```python
from build123d import *

# Parameters (mm, degrees)
BOSS_EXTRUDE1_DEPTH     = 56
SKETCH2_R               = 20
BOSS_EXTRUDE2_DEPTH     = 2
SKETCH4_R               = 20
BOSS_EXTRUDE3_DEPTH     = 2
SKETCH5_R               = 2.5
CUT_EXTRUDE1_DEPTH      = 11
SKETCH6_R               = 2.5
CUT_EXTRUDE2_DEPTH      = 11
CUT_EXTRUDE3_DEPTH      = 147.710599481
CUT_EXTRUDE3_DEPTH_BACK = 147.710599481
SKETCH7_R               = 11
SKETCH8_R               = 11
CUT_EXTRUDE4_DEPTH      = 51


with BuildPart() as part:
    # Sketch1 → Boss-Extrude1 (new body)
    with BuildSketch(Plane.XY):
        Polygon((-52, 0), (52, 0), (52, -56), (28, -56), (28, -80), (-28, -80), (-28, -56), (-52, -56), align=None)
    extrude(amount=BOSS_EXTRUDE1_DEPTH)

    # Sketch2 → Boss-Extrude2 (add)
    with BuildSketch(Plane(origin=(52, 0, 0), x_dir=(0, 0, -1), z_dir=(1, 0, 0))):
        with Locations(Location((-28, -28, 0), (0, 0, 90))):
            Circle(SKETCH2_R)
    boss_extrude2 = extrude(amount=BOSS_EXTRUDE2_DEPTH)

    # Mirror1: Boss-Extrude2 across plane
    add(boss_extrude2.mirror(Plane(origin=(0, 0, 0), x_dir=(0, 0, 1), z_dir=(1, 0, 0))))

    # Sketch4 → Boss-Extrude3 (add)
    with BuildSketch(Plane.XZ.offset(80)):
        with Locations(Location((0, 28, 0), (0, 0, 270))):
            Circle(SKETCH4_R)
    extrude(amount=BOSS_EXTRUDE3_DEPTH)

    # Sketch5 → Cut-Extrude1 (cut)
    with BuildSketch(Plane(origin=(52, 0, 0), x_dir=(0, 0, -1), z_dir=(1, 0, 0))):
        with Locations(Location((-50, -6, 0), (0, 0, 90))):
            Circle(SKETCH5_R)
        with Locations(Location((-50, -50, 0), (0, 0, 90))):
            Circle(SKETCH5_R)
        with Locations(Location((-6, -50, 0), (0, 0, 90))):
            Circle(SKETCH5_R)
        with Locations(Location((-6, -6, 0), (0, 0, 90))):
            Circle(SKETCH5_R)
    cut_extrude1 = extrude(amount=-CUT_EXTRUDE1_DEPTH, mode=Mode.SUBTRACT)

    # Mirror2: Cut-Extrude1 across plane
    add(cut_extrude1.mirror(Plane(origin=(0, 0, 0), x_dir=(0, 0, 1), z_dir=(1, 0, 0))), mode=Mode.SUBTRACT)

    # Sketch6 → Cut-Extrude2 (cut)
    with BuildSketch(Plane.XZ.offset(80)):
        with Locations(Location((-22, 50, 0), (0, 0, 270))):
            Circle(SKETCH6_R)
        with Locations(Location((22, 50, 0), (0, 0, 270))):
            Circle(SKETCH6_R)
        with Locations(Location((22, 6, 0), (0, 0, 270))):
            Circle(SKETCH6_R)
        with Locations(Location((-22, 6, 0), (0, 0, 270))):
            Circle(SKETCH6_R)
    extrude(amount=-CUT_EXTRUDE2_DEPTH, mode=Mode.SUBTRACT)

    # Sketch7 → Cut-Extrude3 (cut, two sides: drawn at the far end of the back side and taken through both)
    with BuildSketch(Plane.ZY.offset(54).offset(-CUT_EXTRUDE3_DEPTH_BACK)):
        with Locations(Location((28, -28, 0), (0, 0, 270))):
            Circle(SKETCH7_R)
    extrude(amount=CUT_EXTRUDE3_DEPTH + CUT_EXTRUDE3_DEPTH_BACK, mode=Mode.SUBTRACT)

    # Sketch8 → Cut-Extrude4 (cut)
    with BuildSketch(Plane.XZ.offset(82)):
        with Locations(Location((0, 28, 0), (0, 0, 270))):
            Circle(SKETCH8_R)
    extrude(amount=-CUT_EXTRUDE4_DEPTH, mode=Mode.SUBTRACT)


solid = part.part
```
For this review, take the finished solid that the model builds, in its own axes (mm). A direction names the side the tool comes from. Round coordinates to 2 decimals unless told otherwise and drop trailing zeros. Write each loop counter-clockwise with the first axis right and the second up, starting at its lowest first coordinate (ties: lowest second). Pieces come first, ordered by that corner, then holes. Notation, with made-up numbers: (10, 45) -> (27, 45) arc R15 ccw to (27, 70) -> close; hole circle Ø9 at (71.25, 20). An arc over 180 degrees is marked (long way). Use one line per item in the form item = value.
Q1. The part is to be moulded in two halves that separate along X. For faces 1 (the flat face through (52, -21, 9)), 2 (the flat face through (-52, -47, 21)), 3 (the cylindrical face through (24.11, -74.58, 4.66)), say which applies: released by +X, released by -X, zero draft, split by the parting line, or undercut.
Resolved:
face_1 = released by +X
face_2 = released by -X
face_3 = undercut
Q2. Consider section B-B (y = -50). State the section outline as (x, z) points.
Resolved:
outline = (-52, 0) -> (52, 0) -> (52, 3.5) -> (41, 3.5) -> (41, 8.5) -> (52, 8.5) -> (52, 47.5) -> (41, 47.5) -> (41, 52.5) -> (52, 52.5) -> (52, 56) -> (-52, 56) -> (-52, 52.5) -> (-41, 52.5) -> (-41, 47.5) -> (-52, 47.5) -> (-52, 8.5) -> (-41, 8.5) -> (-41, 3.5) -> (-52, 3.5) -> close; hole circle Ø22 at (0, 28)
Q3. Consider section A-A (x = -22). State the section outline as (y, z) points.
Resolved:
outline = (-80, 0) -> (0, 0) -> (0, 56) -> (-80, 56) -> (-80, 52.5) -> (-69, 52.5) -> (-69, 47.5) -> (-80, 47.5) -> (-80, 8.5) -> (-69, 8.5) -> (-69, 3.5) -> (-80, 3.5) -> close; hole circle Ø22 at (-28, 28)
Q4. Consider section D-D (y = -28). State the section outline as (x, z) points, then the cut area to 3 significant figures.
Resolved:
outline = (-54, 8) -> (-52, 8) -> (-52, 0) -> (52, 0) -> (52, 8) -> (54, 8) -> (54, 17) -> (-54, 17) -> close; (-54, 39) -> (54, 39) -> (54, 48) -> (52, 48) -> (52, 56) -> (-52, 56) -> (-52, 48) -> (-54, 48) -> close
area = 3,610 mm²
Q5. Consider section C-C (z = 21). State the section outline as (x, y) points (3 decimals).
Resolved:
outline = (-54, -46.735) -> (-52, -46.735) -> (-52, -56) -> (-28, -56) -> (-28, -80) -> (-18.735, -80) -> (-18.735, -82) -> (-8.485, -82) -> (-8.485, -36.485) -> (-54, -36.485) -> close; (-54, -19.515) -> (54, -19.515) -> (54, -9.265) -> (52, -9.265) -> (52, 0) -> (-52, 0) -> (-52, -9.265) -> (-54, -9.265) -> close; (8.485, -82) -> (18.735, -82) -> (18.735, -80) -> (28, -80) -> (28, -56) -> (52, -56) -> (52, -46.735) -> (54, -46.735) -> (54, -36.485) -> (8.485, -36.485) -> close
Q6. Clearance check with flat-ended pins moving along their axes: pin 1 Ø8 at (x, z) = (22, 6) entering from -Y; pin 2 Ø17 at (y, z) = (-28.5, 20) entering from -X; pin 3 Ø20 at (x, z) = (0, 28) entering from -Y; pin 4 Ø4 at (y, z) = (-52.5, 30.5) entering from +X. State where each tip first meets the part, or that it passes through.
Resolved:
pin_1 = -80
pin_2 = -54
pin_3 = -23.42
pin_4 = 52
Q7. To check wall thickness, follow probe 1 along X at (y, z) = (-73, 6); probe 2 along Z at (x, y) = (-47.75, -50); probe 3 along Z at (x, y) = (0, -51). State the ranges of each line that lie inside material, in increasing order. Write a range as from..to.
Resolved:
probe_1 = -28..-24.5, -19.5..19.5, 24.5..28
probe_2 = 0..3.5, 8.5..47.5, 52.5..56
probe_3 = 0..17, 39..56
Q8. Machinability: for faces 4 (the cylindrical face through (24.11, -74.58, 48.66)), 5 (the flat face through (-28, -68, 28)), 6 (the flat face through (41, -6, 6)), 7 (the cylindrical face through (-46.577, -47.615, 6.751)), 8 (the flat face through (-54, -19, 19)), which of the approach directions +Z, -Z, +X, -X, +Y, -Y give a long, thin tool a straight path to every point of the face, cutting with its end or side? Answer none if there is none.
Resolved:
face_4 = -Y
face_5 = +Z, -Z, -X, -Y
face_6 = +X
face_7 = -X
face_8 = +Z, -Z, -X, +Y, -Y
